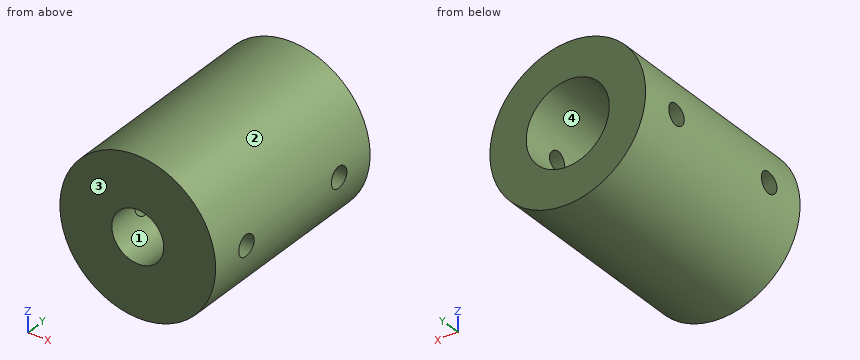
from build123d import *

# Parameters (mm, degrees)
SKETCH1_R               = 7.5
SKETCH1_R_2             = 4
BOSS_EXTRUDE2_DEPTH     = 10
BOSS_EXTRUDE3_START     = -10
SKETCH1_3_R             = 7.5
SKETCH1_3_R_2           = 4
SKETCH1_3_R_3           = 2.5
BOSS_EXTRUDE3_DEPTH     = 10
CUT_EXTRUDE1_DEPTH      = 15.577379737
CUT_EXTRUDE1_DEPTH_BACK = 15.577379737
SKETCH2_R               = 1


with BuildPart() as part:
    # Sketch1 → Boss-Extrude2 (new body)
    with BuildSketch(Plane(origin=(0, 0, 0), x_dir=(1, 0, 0), z_dir=(0, 1, 0))):
        with Locations(Location((0, 0, 0), (0, 0, 270))):
            Circle(SKETCH1_R)
        with Locations(Location((0, 0, 0), (0, 0, 270))):
            Circle(SKETCH1_R_2, mode=Mode.SUBTRACT)
    extrude(amount=BOSS_EXTRUDE2_DEPTH)

    # Sketch1_3 → Boss-Extrude3 (add)
    # profile 1 of 2: a face of its own
    with BuildSketch(Plane(origin=(0, 0, 0), x_dir=(1, 0, 0), z_dir=(0, 1, 0)).offset(BOSS_EXTRUDE3_START)):
        with Locations(Location((0, 0, 0), (0, 0, 270))):
            Circle(SKETCH1_3_R)
        with Locations(Location((0, 0, 0), (0, 0, 270))):
            Circle(SKETCH1_3_R_2, mode=Mode.SUBTRACT)
    # profile 2 of 2: a face of its own
    with BuildSketch(Plane(origin=(0, 0, 0), x_dir=(1, 0, 0), z_dir=(0, 1, 0)).offset(BOSS_EXTRUDE3_START)):
        with Locations(Location((0, 0, 0), (0, 0, 270))):
            Circle(SKETCH1_3_R_2)
        with Locations(Location((0, 0, 0), (0, 0, 270))):
            Circle(SKETCH1_3_R_3, mode=Mode.SUBTRACT)
    extrude(amount=BOSS_EXTRUDE3_DEPTH)

    # Sketch2 → Cut-Extrude1 (cut, two sides: drawn at the far end of the back side and taken through both)
    with BuildSketch(Plane(origin=(0, 0, 0), x_dir=(0, 0, -1), z_dir=(1, 0, 0)).offset(-CUT_EXTRUDE1_DEPTH_BACK)):
        with Locations((0, 6)):
            Circle(SKETCH2_R)
        with Locations((0, -6)):
            Circle(SKETCH2_R)
    extrude(amount=CUT_EXTRUDE1_DEPTH + CUT_EXTRUDE1_DEPTH_BACK, mode=Mode.SUBTRACT)


solid = part.part
Here's how the part is built. I have some questions about the finished solid (model axes, mm). Face numbers are marked on the shaded views. Coordinates: 2 decimals unless noted, no trailing zeros. Write each loop counter-clockwise with the first axis right and the second up, starting at its lowest first coordinate (ties: lowest second). Pieces come first, ordered by that corner, then holes.
Item 1: Will these pins go through, and if not, where does the flat tip stop? pin 1 (6.5 mm diameter, centred on x = 0.5, z = -0.5, fed in from +Y); pin 2 (4 mm diameter, centred on y = 2.5, z = 1.5, fed in from -X); pin 3 (2 mm diameter, centred on y = 8, z = 4.5, fed in from +X).
Item 2: I want a section at D-D on y = 3.25. Write out the boundary of the cut face in (x, z).
Item 3: If we mould it in two halves opening along X, with no side actions, what happens to the marked faces 1, 2, 3 and 4? For each: +X half, -X half, draft (parallel to the pull), parting line (faces both ways), or undercut.
Item 4: If I drill on line 1 (X direction, y = 3.25, z = 0); line 2 (Y direction, x = 2.75, z = 2.5); line 3 (Z direction, x = -3.6, y = -6), over which ranges is the centre line in solid material (lowest first)?
Item 5: I want a section at C-C on z = 0.75. Write out the boundary of the cut face in (x, y), and give its area (3 significant figures).
Item 6: I want a section at B-B on y = 6. Write out the boundary of the cut face in (x, z).
Item 7: I want a section at A-A on x = 0. Write out the boundary of the cut face in (y, z), and give its area (3 significant figures).
Findings below:
1. pin 1: stops at y = 0
1. pin 2: stops at x = -7.5
1. pin 3: stops at x = 6.63
2. outline: circle Ø15 at (0, 0); hole circle Ø8 at (0, 0)
3. face 1: undercut
3. face 2: parting line
3. face 3: draft
3. face 4: undercut
4. line 1: x = -7.5 to -4, 4 to 7.5
4. line 2: y = -10 to 0
4. line 3: z = -6.58 to -1, 1 to 6.58
5. outline: (-7.46, -10) - (-2.38, -10) - (-2.38, -6.66) - (-7.46, -6.66) - close; (-7.46, -5.34) - (-2.38, -5.34) - (-2.38, 0) - (-3.93, 0) - (-3.93, 5.34) - (-7.46, 5.34) - close; (-7.46, 6.66) - (-3.93, 6.66) - (-3.93, 10) - (-7.46, 10) - close; (2.38, -10) - (7.46, -10) - (7.46, -6.66) - (2.38, -6.66) - close; (2.38, -5.34) - (7.46, -5.34) - (7.46, 5.34) - (3.93, 5.34) - (3.93, 0) - (2.38, 0) - close; (3.93, 6.66) - (7.46, 6.66) - (7.46, 10) - (3.93, 10) - close
5. area: 149 mm2
6. outline: (-7.43, -1) arc R7.5 ccw to (7.43, -1) - (3.87, -1) arc R4 cw to (-3.87, -1) - close; (-7.43, 1) - (-3.87, 1) arc R4 cw to (3.87, 1) - (7.43, 1) arc R7.5 ccw to start
7. outline: (-10, -7.5) - (10, -7.5) - (10, -4) - (0, -4) - (0, -2.5) - (-10, -2.5) - close; (-10, 2.5) - (0, 2.5) - (0, 4) - (10, 4) - (10, 7.5) - (-10, 7.5) - close
7. area: 170 mm2
